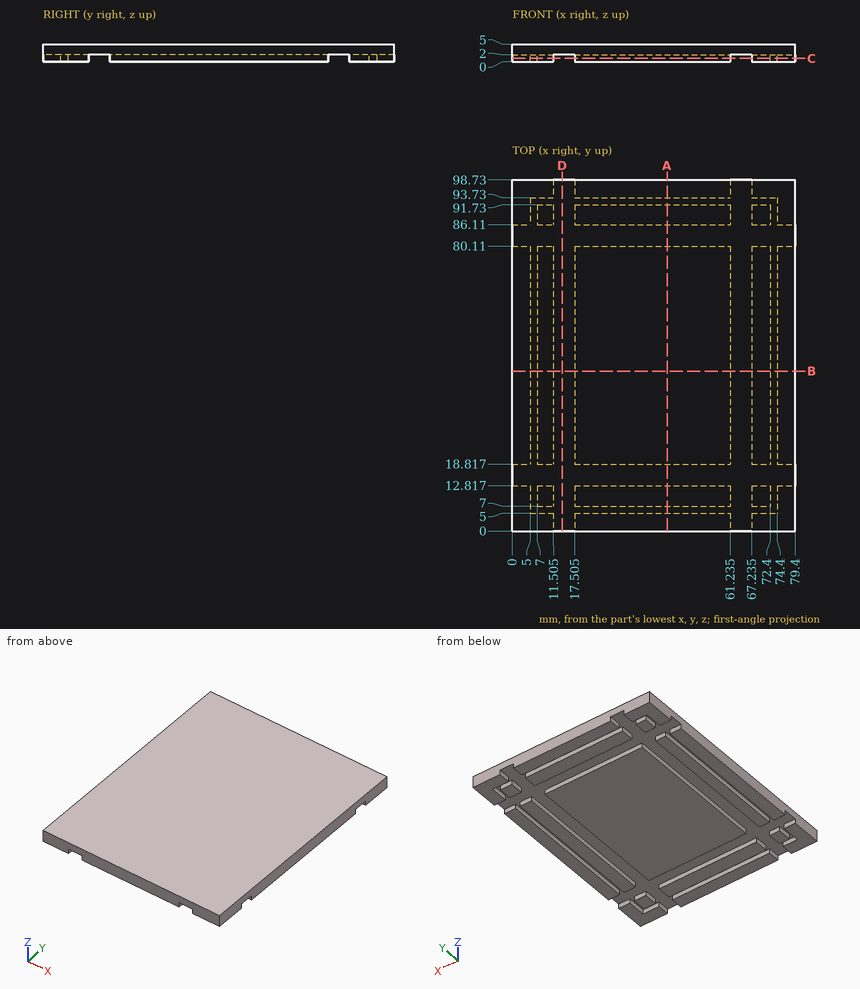
Verification items for this drawing (mm, ordinates from the low corner). Coordinates: 2 decimals unless noted, no trailing zeros. Order: outer loops, then holes, each group sorted by start corner. A loop starts at its lowest first (then second) coordinate and runs counter-clockwise, first axis right, second up. Notation, with made-up numbers: (24.5, 54.25) -> (67.5, 54.25) arc R21 cw to (67.5, 61.25) -> close; hole circle Ø10 at (28, -11). An arc over 180 degrees is marked (long way). Put each result on its own line as item: value. Start each with the question number.
1. Cross-section at C-C, the plane z = 0.95. Count the separate pieces of the cut face and the enclosed holes in it.
2. Cross-section at D-D, the plane x = 14. Record the boundary of the cut face in (y, z).
3. Go/stop test with a flat-tipped pin: pin 1 Ø1 at (x, y) = (65, 29) entering from -Z. Record where the tip stops, or that it passes through.
4. Cross-section at B-B, the plane y = 45. Record the boundary of the cut face in (x, z) (1 decimal).
5. Cross-section at A-A, the plane x = 43.5. Record the boundary of the cut face in (y, z).
6. Material ranges on L1, parallel to Y at x = 56, z = 1.65; L2, parallel to X at y = 56.5, z = 0.4 (1 decimal); L3, parallel to Y at x = 5.5, z = 0.5, recorded low to high. Write a range as [from, to].
Computed:
1. separate pieces: 17
1. enclosed holes: 0
2. outline: (0, 2) -> (98.73, 2) -> (98.73, 5) -> (0, 5) -> close
3. pin 1: z = 2
4. outline: (0, 0) -> (5, 0) -> (5, 2) -> (7, 2) -> (7, 0) -> (11.5, 0) -> (11.5, 2) -> (17.5, 2) -> (17.5, 0) -> (61.2, 0) -> (61.2, 2) -> (67.2, 2) -> (67.2, 0) -> (72.4, 0) -> (72.4, 2) -> (74.4, 2) -> (74.4, 0) -> (79.4, 0) -> (79.4, 5) -> (0, 5) -> close
5. outline: (0, 0) -> (5, 0) -> (5, 2) -> (7, 2) -> (7, 0) -> (12.82, 0) -> (12.82, 2) -> (18.82, 2) -> (18.82, 0) -> (80.11, 0) -> (80.11, 2) -> (86.11, 2) -> (86.11, 0) -> (91.73, 0) -> (91.73, 2) -> (93.73, 2) -> (93.73, 0) -> (98.73, 0) -> (98.73, 5) -> (0, 5) -> close
6. L1: [0, 5], [7, 12.82], [18.82, 80.11], [86.11, 91.73], [93.73, 98.73]
6. L2: [0, 5], [7, 11.5], [17.5, 61.2], [67.2, 72.4], [74.4, 79.4]
6. L3: [0, 5], [93.73, 98.73]
